Could you check a few things on this model? Use its own coordinates, in mm. A direction names the side the tool comes from. Round coordinates to 2 decimals unless told otherwise and drop trailing zeros. Loops run counter-clockwise (first coordinate to the right, second up) from the corner with the lowest first, then second, coordinate; pieces in that order, holes last. Notation, with made-up numbers: M -2,77 L 18,77 A4 cw 18,82 Z; hole C 52.25,85.5 d4. An arc over 180 degrees is marked long. One line per item, written item: value. Start each with the question number.
Q1. Imagine slicing it at C-C (z = 39). Please give me the cut outline in (x, y), then the cut area to 3 significant figures.
Q2. Imagine slicing it at D-D (x = -23.55). Please give me the cut outline in (y, z).
Q3. I'm going to push flat-ended pins straight in: pin 1 Ø8 at (x, z) = (-23.55, 62.55) entering from -Y; pin 2 Ø4.5 at (x, z) = (23.55, 15.45) entering from +Y; pin 3 Ø19 at (x, z) = (-16, 44) entering from +Y; pin 4 Ø1 at (x, y) = (25.5, 52.5) entering from +Z. Where does each tip first touch, or does it pass through?
Q4. Which directions (+Z, -Z, +X, -X, +Y, -Y) give clear straight access to the entire face, cutting with the end or side of a thin tool? Please do faces 5 (the face through (29.5, 8, 11)), 6 (the face through (-22.15, 37, 1)), 7 (the face through (0, 68, 1)).
Q5. Imagine slicing it at A-A (x = 20). Please give me the cut outline in (y, z), then the cut area to 3 significant figures.
Q6. Please list where these lines run through material, in increasing order: line 1 along Z through (x, y) = (23, 1); line 2 along X through (y, z) = (2, 15); line 3 along Z through (x, y) = (1.5, 15).
Q7. Imagine slicing it at B-B (y = 46.5). Please give me the cut outline in (x, z).
Q8. Thinking about a two-plate mould opening in Y: for faces 1 (the face through (0, 1, 2)), 2 (the face through (-25.534, 1.479, 13.929)), 3 (the face through (-20, 14, 1)), 4 (the face through (31.02, 11.62, 16.31)), which applies, released by +Y, released by -Y, zero draft, split by the parting line, or undercut?
from build123d import *

# Parameters (mm, degrees)
F1_DEPTH  = 32.5
F2_R      = 5
F3_R      = 2
F4_R      = 19.05
F4_R_2    = 2.5
F5_DEPTH  = 68.001
F7_DEPTH  = 68.001
F9_DEPTH  = 3
F11_DEPTH = 3
F12_SIZE  = 5


with BuildPart() as f1:
    # F0 (on Right) → F1 (new body, symmetric)
    with BuildSketch(Plane.YZ):
        Polygon((0, 68), (0, 0), (68, 0), (68, 3), (3, 3), (3, 68), align=None)
    extrude(amount=F1_DEPTH, both=True)

    # F2
    f2_edges = [f1.edges().sort_by_distance(p)[0] for p in [
        (0, 0, 0),
    ]]
    fillet(f2_edges, radius=F2_R)

    # F3
    f3_edges = [f1.edges().sort_by_distance(p)[0] for p in [
        (0, 3, 3),
    ]]
    fillet(f3_edges, radius=F3_R)

    # F4 (on face) → F5 (cut, through all)
    with BuildSketch(Plane.XZ):
        with Locations((0, 39)):
            Circle(F4_R)
        with Locations((-23.55, 15.45)):
            Circle(F4_R_2)
        with Locations((23.55, 15.45)):
            Circle(F4_R_2)
        with Locations((23.55, 62.55)):
            Circle(F4_R_2)
        with Locations((-23.55, 62.55)):
            Circle(F4_R_2)
    extrude(amount=-F5_DEPTH, mode=Mode.SUBTRACT)

    # F6 (on face) → F7 (cut, through all)
    with BuildSketch(Plane(origin=(0, 0, 0), x_dir=(1, 0, 0), z_dir=(0, 0, -1))):
        with BuildLine():
            ThreePointArc((-22.15, -57.85), (-20, -60), (-17.85, -57.85))
            Line((-17.85, -57.85), (-17.85, -16.15))
            ThreePointArc((-17.85, -16.15), (-20, -14), (-22.15, -16.15))
            Line((-22.15, -16.15), (-22.15, -57.85))
        make_face()
        with BuildLine():
            ThreePointArc((17.85, -57.85), (20, -60), (22.15, -57.85))
            Line((22.15, -57.85), (22.15, -16.15))
            ThreePointArc((22.15, -16.15), (20, -14), (17.85, -16.15))
            Line((17.85, -16.15), (17.85, -57.85))
        make_face()
    extrude(amount=-F7_DEPTH, mode=Mode.SUBTRACT)

    # F8 (on face) → F9 (join)
    with BuildSketch(Plane.YZ.offset(32.5)):
        with BuildLine():
            Line((3, 30), (3, 5))
            ThreePointArc((3, 5), (3.585786, 3.585786), (5, 3))
            Line((5, 3), (20, 3))
            Line((20, 3), (3, 30))
        make_face()
    extrude(amount=-F9_DEPTH)

    # F10 (on face) → F11 (join)
    with BuildSketch(Plane(origin=(-32.5, 0, 0), x_dir=(0, -1, 0), z_dir=(-1, 0, 0))):
        with BuildLine():
            Line((-3, 5), (-3, 30))
            Line((-3, 30), (-20, 3))
            Line((-20, 3), (-5, 3))
            ThreePointArc((-5, 3), (-3.585786, 3.585786), (-3, 5))
        make_face()
    extrude(amount=-F11_DEPTH)

    # F12
    f12_edges = [f1.edges().sort_by_distance(p)[0] for p in [
        (32.5, 1.5, 68),
        (32.5, 68, 1.5),
        (-32.5, 68, 1.5),
        (-32.5, 1.5, 68),
    ]]
    chamfer(f12_edges, length=F12_SIZE)


solid = f1.part
Report:
1. outline: M -32.5,0 L -19.05,0 L -19.05,3 L -32.5,3 Z; M 19.05,0 L 32.5,0 L 32.5,3 L 19.05,3 Z
1. area: 80.7 mm²
2. outline: M 0,5 A5 ccw 5,0 L 68,0 L 68,3 L 5,3 A2 cw 3,5 L 3,12.95 L 0,12.95 Z; M 0,17.95 L 3,17.95 L 3,60.05 L 0,60.05 Z; M 0,65.05 L 3,65.05 L 3,68 L 0,68 Z
3. pin 1: stops at y = 0
3. pin 2: passes through
3. pin 3: stops at y = 3
3. pin 4: stops at z = 3
4. face 5: +Z, +Y
4. face 6: +Z, -Z
4. face 7: +Z, -Z, +X, -X, +Y
5. outline: M 0,5 A5 ccw 5,0 L 14,0 L 14,3 L 5,3 A2 cw 3,5 L 3,68 L 0,68 Z; M 60,0 L 68,0 L 68,3 L 60,3 Z
5. area: 256 mm²
6. line 1: z = 2 to 13.01, 17.89 to 60.11, 64.99 to 68
6. line 2: x = -32.5 to -26.01, -21.09 to 21.09, 26.01 to 32.5
6. line 3: z = 0 to 3
7. outline: M -32.5,0 L -22.15,0 L -22.15,3 L -32.5,3 Z; M -17.85,0 L 17.85,0 L 17.85,3 L -17.85,3 Z; M 22.15,0 L 32.5,0 L 32.5,3 L 22.15,3 Z
8. face 1: released by -Y
8. face 2: zero draft
8. face 3: undercut
8. face 4: released by +Y
